Answer from the drawing. Dimensions are ordinates in mm from the lowest x, y and z of the part. Round coordinates to 2 decimals unless told otherwise and drop trailing zeros. Loops run counter-clockwise (first coordinate to the right, second up) from the corner with the lowest first, then second, coordinate; pieces in that order, holes last. Notation, with made-up numbers: M 21.5,18 L 54.5,18 A30 ccw 54.5,55 Z; hole C 4.25,9.5 d6. An arc over 180 degrees is marked long. Write each question's results on one line, items separated by ' | '.
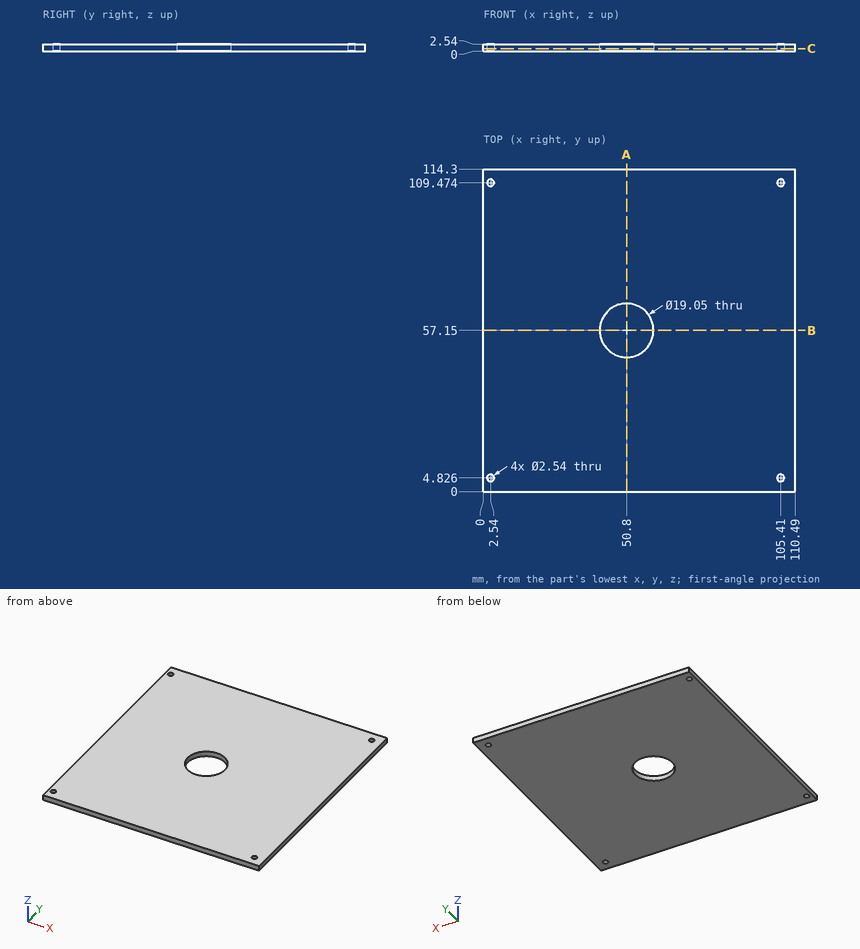
1. Find section B-B, the plane y = 57.15. Give the vertices of the cut face in (x, z) (3 decimals), then the cut area to 3 significant figures.
Completed:
outline: M 0,0 L 41.275,0 L 41.275,2.54 L 0,2.54 Z; M 60.325,0 L 110.49,0 L 110.49,2.54 L 60.325,2.54 Z | area: 232 mm2
2. Find the intervals of material crossed by L1, parallel to X at y = 56.5, z = 1.7; L2, parallel to Y at x = 53, z = 1.7; L3, parallel to Y at x = 58, z = 1.2, in increasing order.
Completed:
L1: x = 0 to 41.3, 60.3 to 110.49 | L2: y = 0 to 47.88, 66.42 to 114.3 | L3: y = 0 to 50.91, 63.39 to 114.3
3. Given P1, Ø10, axis at x = 25, y = 80.5, coming from the -Z side, flat-ended and moving along its own axis, determine where the tip first touches the part or whether it passes through.
Completed:
P1: stops at z = 0
4. Find section A-A, the plane x = 50.8. Give the vertices of the cut face in (y, z) (3 decimals).
Completed:
outline: M 0,0 L 47.625,0 L 47.625,2.54 L 0,2.54 Z; M 66.675,0 L 114.3,0 L 114.3,2.54 L 66.675,2.54 Z
5. Find section C-C, the plane z = 0.9. Give the vertices of the cut face in (x, y) (3 decimals).
Completed:
outline: M 0,0 L 110.49,0 L 110.49,114.3 L 0,114.3 Z; hole C 2.54,4.826 d2.54; hole C 2.54,109.474 d2.54; hole C 50.8,57.15 d19.05; hole C 105.41,4.826 d2.54; hole C 105.41,109.474 d2.54
